Source: CAD feature listing. Evaluate the final solid. Frame: model axes, mm. A direction names the side the tool comes from. Give positions to 0.01 mm unless a question says otherwise; leave off trailing zeros. Loops run counter-clockwise (first coordinate to the right, second up) from the corner with the lowest first, then second, coordinate; pieces in that order, holes last.
from build123d import *

# Parameters (mm, degrees)
BOSS_EXTRUDE1_DEPTH        = 2.5
SKETCH2_W                  = 15
SKETCH2_H                  = 23.5
BOSS_EXTRUDE2_DEPTH        = 23.5
SKETCH3_W                  = 17.5
SKETCH3_H                  = 23.5
BOSS_EXTRUDE3_DEPTH        = 4.5
SKETCH4_W                  = 17.5
SKETCH4_H                  = 28
BOSS_EXTRUDE4_DEPTH        = 4.5
SKETCH5_W                  = 15
SKETCH5_H                  = 23.5
CUT_EXTRUDE1_DEPTH         = 23.5
BOSS_EXTRUDE5_DEPTH        = 2.5
M3_5_CLEARANCE_HOLE1_D     = 4.134
M3_5_CLEARANCE_HOLE1_DEPTH = 2.5
F_6_3_6_3_DIAMETER_HOLE1_D = 6.3
F_6_3_6_3_DIAMETER_HOLE2_D = 6.3
M3_5_CLEARANCE_HOLE2_D     = 4.134
M3_5_CLEARANCE_HOLE2_DEPTH = 20
CHAMFER1_SIZE              = 0.433
FILLET2_START              = -11
FILLET2_DEPTH              = 22


with BuildPart() as part:
    # Sketch1 → Boss-Extrude1 (new body)
    with BuildSketch(Plane(origin=(-10, 0, 0), x_dir=(0, -1, 0), z_dir=(-1, 0, 0))):
        with BuildLine():
            Line((-27.707106781, 4.792893219), (-28, 4.5))
            Line((-28, 4.5), (-4.5, 4.5))
            Line((-4.5, 4.5), (-4.5, 28))
            Line((-4.5, 28), (-4.792893219, 27.707106781))
            add(Edge.make_bspline(
                [(-4.792893219, 27.707106781), (-12.430964406, 20.069035594), (-20.069035594, 12.430964406), (-27.707106781, 4.792893219)],
                knots=[0, 0, 0, 0, 1, 1, 1, 1], degree=3))
        make_face()
    extrude(amount=-BOSS_EXTRUDE1_DEPTH)

    # Sketch2 → Boss-Extrude2 (add)
    with BuildSketch(Plane.XZ.offset(-4.5)):
        with Locations((0, 16.25)):
            Rectangle(SKETCH2_W, SKETCH2_H)
    extrude(amount=-BOSS_EXTRUDE2_DEPTH)

    # Sketch3 → Boss-Extrude3 (add)
    with BuildSketch(Plane(origin=(0, 0, 4.5), x_dir=(-1, 0, 0), z_dir=(0, 0, -1))):
        with Locations((1.25, 16.25)):
            Rectangle(SKETCH3_W, SKETCH3_H)
    extrude(amount=BOSS_EXTRUDE3_DEPTH)

    # Sketch4 → Boss-Extrude4 (add)
    with BuildSketch(Plane.XZ.offset(-4.5)):
        with Locations((-1.25, 14)):
            Rectangle(SKETCH4_W, SKETCH4_H)
    extrude(amount=BOSS_EXTRUDE4_DEPTH)

    # Sketch5 → Cut-Extrude1 (cut)
    with BuildSketch(Plane(origin=(0, 28, 0), x_dir=(-1, 0, 0), z_dir=(0, 1, 0))):
        with Locations((0, 16.25)):
            Rectangle(SKETCH5_W, SKETCH5_H)
    extrude(amount=-CUT_EXTRUDE1_DEPTH, mode=Mode.SUBTRACT)

    # Sketch6 → Boss-Extrude5 (add)
    with BuildSketch(Plane(origin=(7.5, 0, 0), x_dir=(0, 0, -1), z_dir=(1, 0, 0))):
        with BuildLine():
            Line((-28, 0), (-28, 4.5))
            Line((-28, 4.5), (-27.707106781, 4.792893219))
            add(Edge.make_bspline(
                [(-4.792893219, 27.707106781), (-12.430964406, 20.069035594), (-20.069035594, 12.430964406), (-27.707106781, 4.792893219)],
                knots=[0, 0, 0, 0, 1, 1, 1, 1], degree=3))
            Line((-4.792893219, 27.707106781), (-4.5, 28))
            Line((-4.5, 28), (0, 28))
            Line((0, 28), (0, 0))
            Line((0, 0), (-28, 0))
        make_face()
    extrude(amount=BOSS_EXTRUDE5_DEPTH)

    # M3.5 Clearance Hole1
    with Locations(Plane.ZY.offset(-7.5)):
        with Locations((12, 12)):
            Hole(M3_5_CLEARANCE_HOLE1_D / 2, depth=M3_5_CLEARANCE_HOLE1_DEPTH)

    # Ø6.3 (6.3) Diameter Hole1 (through all)
    with Locations(Plane(origin=(0, 4.5, 0), x_dir=(1, 0, 0), z_dir=(0, 1, 0))):
        with Locations((0, -20)):
            Hole(F_6_3_6_3_DIAMETER_HOLE1_D / 2)

    # Ø6.3 (6.3) Diameter Hole2 (through all)
    with Locations(Plane.XY.offset(4.5)):
        with Locations((0, 20)):
            Hole(F_6_3_6_3_DIAMETER_HOLE2_D / 2)

    # M3.5 Clearance Hole2
    with Locations(Plane.ZY.offset(10)):
        with Locations((12, 12)):
            Hole(M3_5_CLEARANCE_HOLE2_D / 2, depth=M3_5_CLEARANCE_HOLE2_DEPTH)

    # Chamfer1
    chamfer1_edges = [part.edges().sort_by_distance(p)[0] for p in [
        (-7.5, 12, 14.067),
        (-10, 12, 14.067),
        (7.5, 12, 14.067),
        (10, 12, 14.067),
    ]]
    chamfer(chamfer1_edges, length=CHAMFER1_SIZE)

    # Fillet2: read off the stored shape, not the designer's step
    # Fillet2 outline → Fillet2 (cut)
    with BuildSketch(Plane.YZ.offset(FILLET2_START)):
        with BuildLine():
            Line((4.5, 28), (4.085786438, 28))
            ThreePointArc((4.085786438, 28), (4.46846987, 27.923879533), (4.792893219, 27.707106781))
            Line((4.792893219, 27.707106781), (4.5, 28))
        make_face()
        with BuildLine():
            Line((28, 4.5), (27.707106781, 4.792893219))
            ThreePointArc((27.707106781, 4.792893219), (27.923879533, 4.46846987), (28, 4.085786438))
            Line((28, 4.085786438), (28, 4.5))
        make_face()
    extrude(amount=FILLET2_DEPTH, mode=Mode.SUBTRACT)


solid = part.part
1) Reachability of faces 4 (the flat face through (0, 4.5, 16)), 5 (the flat face through (10, 11, 8)) from +Z, -Z, +X, -X, +Y, -Y: full face, straight path, thin tool, end or side. Return the list, or none.
Checks:
face 4: +Z, +Y
face 5: +Z, -Z, +X, +Y, -Y
2) Cut plane B-B (x = 0). Return loops of the section in (y, z), and give its area (3 significant figures).
Checks:
outline: (0, 0) - (16.85, 0) - (16.85, 4.5) - (4.5, 4.5) - (4.5, 16.85) - (0, 16.85) - close; (0, 23.15) - (4.5, 23.15) - (4.5, 27.91) arc R1 ccw to (4.09, 28) - (0, 28) - close; (23.15, 0) - (28, 0) - (28, 4.09) arc R1 ccw to (27.91, 4.5) - (23.15, 4.5) - close
area: 175 mm2
3) Contact query for flat-ended pins moving along their axis: P1, Ø5, axis at x = 0, y = 20, coming from the +Z side; P2, Ø4, axis at x = 4.5, z = 24, coming from the +Y side; P3, Ø1.5, axis at x = 7.5, z = 24, coming from the +Y side; P4, Ø4.5, axis at x = -1, y = 20, coming from the +Z side. Output: stop coordinate, or through.
Checks:
P1: passes through
P2: stops at y = 4.5
P3: stops at y = 9.25
P4: stops at z = 4.5
4) Cut plane A-A (y = 20). Return loops of the section in (x, z), and give its area (3 significant figures).
Checks:
outline: (-10, 0) - (-3.15, 0) - (-3.15, 4.5) - (-7.5, 4.5) - (-7.5, 12.5) - (-10, 12.5) - close; (3.15, 0) - (10, 0) - (10, 12.5) - (7.5, 12.5) - (7.5, 4.5) - (3.15, 4.5) - close
area: 102 mm2
5) Cut plane C-C (z = 12). Return loops of the section in (x, y), and give its area (3 significant figures).
Checks:
outline: (-10, 0) - (10, 0) - (10, 9.5) - (9.57, 9.93) - (7.93, 9.93) - (7.5, 9.5) - (7.5, 4.5) - (-7.5, 4.5) - (-7.5, 9.5) - (-7.93, 9.93) - (-9.57, 9.93) - (-10, 9.5) - close; (-10, 14.5) - (-9.57, 14.07) - (-7.93, 14.07) - (-7.5, 14.5) - (-7.5, 20.5) - (-10, 20.5) - close; (7.5, 14.5) - (7.93, 14.07) - (9.57, 14.07) - (10, 14.5) - (10, 20.5) - (7.5, 20.5) - close
area: 149 mm2
6) Ray query, probe 1 along Z at (x, y) = (0, 2.75); probe 2 along X at (y, z) = (19.5, 9); probe 3 along Z at (x, y) = (4, 12.5). Return the intervals inside material, ascending.
Checks:
probe 1: z = 0 to 16.85, 23.15 to 28
probe 2: x = -10 to -7.5, 7.5 to 10
probe 3: z = 0 to 4.5
7) Pull-direction query (Y, two-part tool) for faces 1 (the flat face through (8.7, 16.1, 16.4)), 2 (the cylindrical face through (-8.74, 10.74, 13.64)), 3 (the flat face through (0, 16, 4.5)); classes: released by +Y, released by -Y, zero draft, split by the parting line, or undercut.
Checks:
face 1: released by +Y
face 2: undercut
face 3: zero draft
